from build123d import *

# Parameters (mm, degrees)
ESQUISSE1_W        = 36
ESQUISSE1_H        = 66
BOSS_EXTRU_1_DEPTH = 18
CONG_1_R           = 2
ESQUISSE2_R        = 1.5
BOSS_EXTRU_2_DEPTH = 10
ESQUISSE3_R        = 2
ESQUISSE3_R_2      = 1.5
BOSS_EXTRU_3_DEPTH = 5


with BuildPart() as part:
    # Esquisse1 → Boss.-Extru.1 (new body)
    with BuildSketch(Plane.XY):
        with Locations((-0.486264987, 10.73553719)):
            Rectangle(ESQUISSE1_W, ESQUISSE1_H)
    extrude(amount=BOSS_EXTRU_1_DEPTH)

    # Congé1
    cong_1_edges = [part.edges().sort_by_distance(p)[0] for p in [
        (17.513735013, 10.73553719, 18),
        (-0.486264987, 43.73553719, 18),
        (-18.486264987, 10.73553719, 18),
        (-0.486264987, 43.73553719, 0),
        (17.513735013, 10.73553719, 0),
        (-0.486264987, -22.26446281, 0),
        (-18.486264987, 10.73553719, 0),
        (-0.486264987, -22.26446281, 18),
        (-18.486264987, 43.73553719, 9),
        (17.513735013, 43.73553719, 9),
        (17.513735013, -22.26446281, 9),
        (-18.486264987, -22.26446281, 9),
    ]]
    fillet(cong_1_edges, radius=CONG_1_R)

    # Esquisse2 → Boss.-Extru.2 (add)
    with BuildSketch(Plane.XZ.offset(22.26446281)):
        with Locations((-7.00866392, 9)):
            Circle(ESQUISSE2_R)
        with Locations((6.036133945, 9)):
            Circle(ESQUISSE2_R)
    extrude(amount=BOSS_EXTRU_2_DEPTH)

    # Esquisse3 → Boss.-Extru.3 (add)
    with BuildSketch(Plane.XZ.offset(22.26446281)):
        with Locations((-7.00866392, 9)):
            Circle(ESQUISSE3_R)
        with Locations((-7.00866392, 9)):
            Circle(ESQUISSE3_R_2, mode=Mode.SUBTRACT)
        with Locations((6.036133945, 9)):
            Circle(ESQUISSE3_R)
        with Locations((6.036133945, 9)):
            Circle(ESQUISSE3_R_2, mode=Mode.SUBTRACT)
    extrude(amount=BOSS_EXTRU_3_DEPTH)


solid = part.part
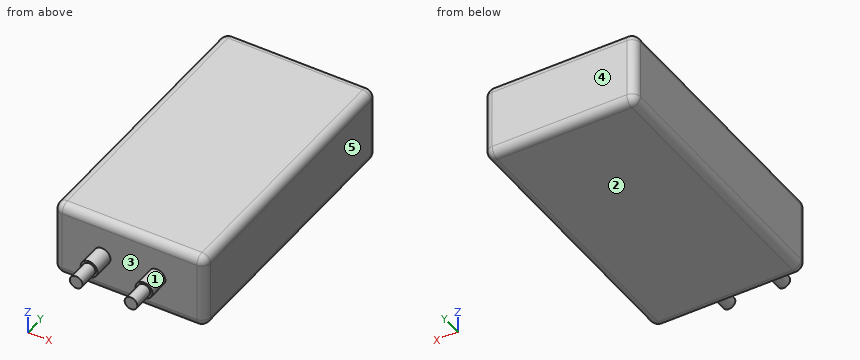
Can you work these out from the model? Positions are in its coordinate system, mm. Face numbers are marked on the shaded views. A direction names the side the tool comes from. Round coordinates to 2 decimals unless told otherwise and drop trailing zeros. Order: outer loops, then holes, each group sorted by start corner. A loop starts at its lowest first (then second) coordinate and runs counter-clockwise, first axis right, second up. Notation, with made-up numbers: M 19,79.25 L 73,79.25 A27 ccw 73,118.25 Z; hole C -37,55.5 d11. An arc over 180 degrees is marked long. Use a Markdown table: item, result.
1) I'm going to push a flat-ended pin straight in: P1, Ø8, axis at x = 11, z = 15.5, coming from the -Y side. Where does the tip first touch, or does it pass through?
Geometry says:
| item | result |
|---|---|
| P1 | stops at y = -22.26 |
2) If I drill on line 1 along X through (y, z) = (17.5, 1.75); line 2 along Y through (x, z) = (7.5, 8.25); line 3 along Y through (x, z) = (-2, 7), over which ranges is the centre line in solid material (lowest first)?
Geometry says:
| item | result |
|---|---|
| line 1 | x = -18.47 to 17.5 |
| line 2 | y = -27.26 to 43.74 |
| line 3 | y = -22.26 to 43.74 |
3) Imagine slicing it at C-C (y = -23.5). List the corners of the cut face in (x, z) for me.
Geometry says:
| item | result |
|---|---|
| outline | C -7.01,9 d4; C 6.04,9 d4 |
4) Imagine slicing it at D-D (z = 9). List the corners of the cut face in (x, y) for me, then the cut area to 3 significant figures.
Geometry says:
| item | result |
|---|---|
| outline | M -18.49,-20.26 A2 ccw -16.49,-22.26 L -9.01,-22.26 L -9.01,-27.26 L -8.51,-27.26 L -8.51,-32.26 L -5.51,-32.26 L -5.51,-27.26 L -5.01,-27.26 L -5.01,-22.26 L 4.04,-22.26 L 4.04,-27.26 L 4.54,-27.26 L 4.54,-32.26 L 7.54,-32.26 L 7.54,-27.26 L 8.04,-27.26 L 8.04,-22.26 L 15.51,-22.26 A2 ccw 17.51,-20.26 L 17.51,41.74 A2 ccw 15.51,43.74 L -16.49,43.74 A2 ccw -18.49,41.74 Z |
| area | 2,440 mm² |
5) Imagine slicing it at B-B (z = 15.25). List the corners of the cut face in (x, y) for me.
Geometry says:
| item | result |
|---|---|
| outline | M -18.49,-20.26 A2 ccw -16.49,-22.26 L 15.51,-22.26 A2 ccw 17.51,-20.26 L 17.51,41.74 A2 ccw 15.51,43.74 L -16.49,43.74 A2 ccw -18.49,41.74 Z |
6) If we mould it in two halves opening along X, with no side actions, what happens to the marked faces 3, 4 and 5? For each: +X half, -X half, draft (parallel to the pull), parting line (faces both ways), or undercut.
Geometry says:
| item | result |
|---|---|
| face 3 | undercut |
| face 4 | draft |
| face 5 | +X half |
7) Imagine slicing it at A-A (x = 14). List the corners of the cut face in (y, z) for me, then the cut area to 3 significant figures.
Geometry says:
| item | result |
|---|---|
| outline | M -22.26,2 A2 ccw -20.26,0 L 41.74,0 A2 ccw 43.74,2 L 43.74,16 A2 ccw 41.74,18 L -20.26,18 A2 ccw -22.26,16 Z |
| area | 1,180 mm² |
8) On a 3-axis mill with a long thin cutter (end or side, diameter ignored), from which of +Z, -Z, +X, -X, +Y, -Y can I reach the whole of each face in a straight line? I mean the marked faces 1 and 2. Say none if no direction works.
Geometry says:
| item | result |
|---|---|
| face 1 | -Y |
| face 2 | -Z, +X, -X, +Y, -Y |
